from build123d import *

# Parameters (mm, degrees)
EXTRUDE_1_DEPTH     = 30
SKETCH_1_W          = 100
SKETCH_1_H          = 100
EXTRUDE_1_2_DEPTH   = 30
SKETCH_2_R          = 7.5
CUT_EXTRUDE_1_DEPTH = 10
CUT_EXTRUDE_2_DEPTH = 190.208879284
SKETCH_4_W          = 100
SKETCH_4_H          = 11.779621946
CUT_EXTRUDE_3_DEPTH = 77.811457479
SKETCH_5_W          = 7.075234897
SKETCH_5_H          = 88.220378054
CUT_EXTRUDE_5_DEPTH = 77.811457479


with BuildPart() as part:
    # Sketch 1 → Extrude 1 (new body)
    with BuildSketch(Plane(origin=(0, 0, 0), x_dir=(1, 0, 0), z_dir=(0, 1, 0))):
        Polygon((80, -50), (180, -50), (80, 50), align=None)
    extrude(amount=EXTRUDE_1_DEPTH)


with BuildPart() as body_2:
    # Sketch 1 → Extrude 1 2 (new body)
    with BuildSketch(Plane(origin=(0, 0, 0), x_dir=(1, 0, 0), z_dir=(0, 1, 0))):
        Rectangle(SKETCH_1_W, SKETCH_1_H)
    extrude(amount=EXTRUDE_1_2_DEPTH)

    # Sketch 2 → Cut-Extrude 1 (cut)
    with BuildSketch(Plane.XZ):
        with Locations(Location((0, 0, 0), (0, 0, 270))):
            Circle(SKETCH_2_R)
        with BuildLine():
            Line((-24.343668286, -22.5), (25.656331714, -22.5))
            ThreePointArc((25.656331714, -22.5), (33.156331714, -30), (25.656331714, -37.5))
            Line((25.656331714, -37.5), (-24.343668286, -37.5))
            ThreePointArc((-24.343668286, -37.5), (-31.843668286, -30), (-24.343668286, -22.5))
        make_face()
    extrude(amount=-CUT_EXTRUDE_1_DEPTH, mode=Mode.SUBTRACT)

    # Sketch 4 → Cut-Extrude 3 (cut, through all)
    with BuildSketch(Plane.XZ):
        with Locations((0, 44.110189027)):
            Rectangle(SKETCH_4_W, SKETCH_4_H)
    extrude(amount=-CUT_EXTRUDE_3_DEPTH, mode=Mode.SUBTRACT)

    # Sketch 5 → Cut-Extrude 5 (cut, through all)
    with BuildSketch(Plane.XZ):
        with Locations((-46.462382551, -5.889810973)):
            Rectangle(SKETCH_5_W, SKETCH_5_H)
    extrude(amount=-CUT_EXTRUDE_5_DEPTH, mode=Mode.SUBTRACT)


with BuildPart() as body_3:
    # Mirror 1: mirrored copy
    add(part.part.mirror(Plane(origin=(0, 0, 0), x_dir=(0, 0, 1), z_dir=(1, 0, 0))))


with BuildPart() as cut_extrude_2_tool:
    # Sketch 3 → Cut-Extrude 2 (new, through all)
    with BuildSketch(Plane.XZ):
        Polygon((80, 50), (80, -50), (180, 50), align=None)
        Polygon((-80, -50), (-80, 50), (-180, 50), align=None)
    extrude(amount=-CUT_EXTRUDE_2_DEPTH)


with BuildPart() as part_1:
    add(part.part)

    # Cut-Extrude 2: cut by cut_extrude_2_tool
    add(cut_extrude_2_tool.part, mode=Mode.SUBTRACT)


with BuildPart() as body_3_1:
    add(body_3.part)

    # Cut-Extrude 2: cut by cut_extrude_2_tool
    add(cut_extrude_2_tool.part, mode=Mode.SUBTRACT)


solid = body_2.part
Source: CAD feature listing. Evaluate the final solid. Frame: model axes, mm. A direction names the side the tool comes from. Give positions to 0.01 mm unless a question says otherwise; leave off trailing zeros. Order: outer loops, then holes, each group sorted by start corner. A loop starts at its lowest first (then second) coordinate and runs counter-clockwise, first axis right, second up. Notation, with made-up numbers: (49, -20.75) -> (90, -20.75) arc R11 ccw to (90, -14.75) -> close; hole circle Ø2 at (2.5, 43). An arc over 180 degrees is marked (long way). Write item = value, one per line.
Q1. Pull-direction query (X, two-part tool) for faces 3 (the face through (0, 10, 0)), 4 (the face through (3, 30, -7)), 5 (the face through (0.33, 4.93, 7.493)), 6 (the face through (-42.925, 15, -7)); classes: released by +X, released by -X, zero draft, split by the parting line, or undercut.
Data:
face_3 = undercut
face_4 = zero draft
face_5 = undercut
face_6 = released by -X
Q2. Cut plane C-C, the plane x = 0. Output: boundary loops of the cut face in (y, z).
Data:
outline = (0, -50) -> (30, -50) -> (30, 38.22) -> (0, 38.22) -> (0, 7.5) -> (10, 7.5) -> (10, -7.5) -> (0, -7.5) -> (0, -22.5) -> (10, -22.5) -> (10, -37.5) -> (0, -37.5) -> close
Q3. Set-up query: faces 1 (the face through (13, 0, -7)), 2 (the face through (33.155, 4.93, -29.835)). Return all of +Z, -Z, +X, -X, +Y, -Y with unobstructed straight access to the full face (end or side cutting, diameter ignored); none if empty.
Data:
face_1 = +Z, -Z, +X, -X, -Y
face_2 = -Y
Q4. Cut plane B-B, the plane x = 11. Output: boundary loops of the cut face in (y, z).
Data:
outline = (0, -50) -> (30, -50) -> (30, 38.22) -> (0, 38.22) -> (0, -22.5) -> (10, -22.5) -> (10, -37.5) -> (0, -37.5) -> close
Q5. Cut plane A-A, the plane z = -30. Output: boundary loops of the cut face in (x, y), and give its area (3 significant figures).
Data:
outline = (-42.92, 0) -> (-31.84, 0) -> (-31.84, 10) -> (33.16, 10) -> (33.16, 0) -> (50, 0) -> (50, 30) -> (-42.92, 30) -> close
area = 2,140 mm^2
Q6. Material intervals for line 1 (X direction, y = 7.5, z = 0); line 2 (Z direction, x = 13, y = 3); line 3 (Z direction, x = -26, y = 8.25), sorted ascending. Write a range as from..to.
Data:
line_1 = -42.92..-7.5, 7.5..50
line_2 = -50..-37.5, -22.5..38.22
line_3 = -50..-37.31, -22.69..38.22
